The drawing under review shows one solid part. Ordinate dimensions are in mm from its lowest x, y, z. A direction names the side the tool comes from. Round coordinates to 2 decimals unless told otherwise and drop trailing zeros. Write each loop counter-clockwise with the first axis right and the second up, starting at its lowest first coordinate (ties: lowest second). Pieces come first, ordered by that corner, then holes. Notation, with made-up numbers: M 41,35.5 L 47,35.5 A6 ccw 47,45.5 Z; hole C 37.25,-29.75 d3. An arc over 180 degrees is marked long. One line per item, written item: value. Start each with the question number.
1) Take a section at C-C, the plane y = 3. Write out the cut boundary in (x, z).
2) Mouldability with a two-part tool opening along Y and no side actions: class the marked faces 4, 5 and 6 as +Y half, -Y half, draft (parallel to the pull), parting line (faces both ways), or undercut.
3) Tool access review of the marked faces 1, 2 and 3: name each direction out of +Z, -Z, +X, -X, +Y, -Y from which nothing blocks a thin tool from reaching the whole face with its end or side.
4) For P1, Ø6.5, axis at x = 7, z = 3.5, coming from the +Y side; P2, Ø3, axis at x = 11.5, y = 5, coming from the +Z side, all flat-tipped, find the tip position at first contact; note any pin that passes through.
5) Take a section at D-D, the plane x = 2. Write out the cut boundary in (y, z).
6) Take a section at B-B, the plane z = 3. Write out the cut boundary in (x, y), and give its area (3 significant figures).
7) Wall thickness on probe 1 along X at (y, z) = (0.35, 3); probe 2 along Z at (x, y) = (16, 1.05); probe 3 along X at (y, z) = (4.4, 12.25): over which ranges is each line inside the solid? List them lowest first.
8) Take a section at A-A, the plane x = 4. Write out the cut boundary in (y, z), and give its area (3 significant figures).
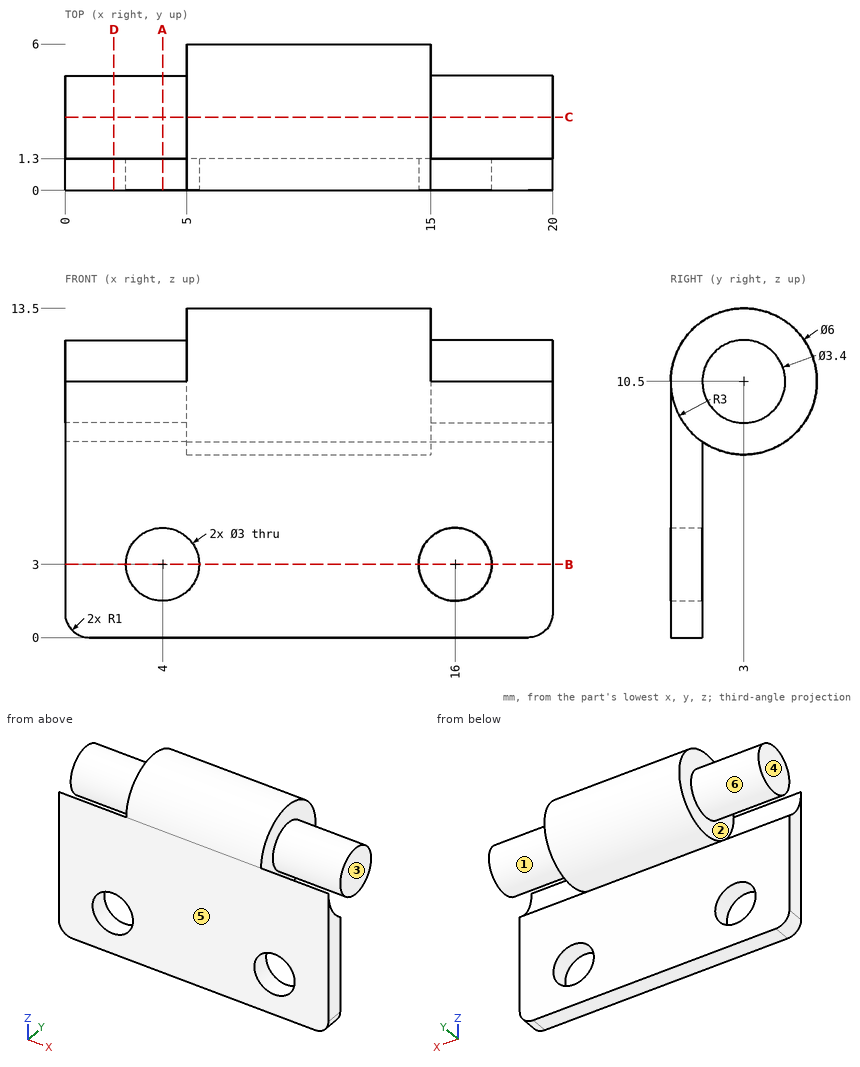
Checked values:
1. outline: M 0,8.8 L 5,8.8 L 5,7.5 L 15,7.5 L 15,8.8 L 20,8.8 L 20,12.2 L 15,12.2 L 15,13.5 L 5,13.5 L 5,12.2 L 0,12.2 Z
2. face 4: draft
2. face 5: -Y half
2. face 6: undercut
3. face 1: +X
3. face 2: -X
3. face 3: +Z, -Z, +X, +Y, -Y
4. P1: stops at y = 1.3
4. P2: stops at z = 13.46
5. outline: M 0,0 L 1.3,0 L 1.3,8.03 A3 cw 0,10.5 Z; C 3,10.5 d3.4
6. outline: M 0,0 L 2.5,0 L 2.5,1.3 L 0,1.3 Z; M 5.5,0 L 14.5,0 L 14.5,1.3 L 5.5,1.3 Z; M 17.5,0 L 20,0 L 20,1.3 L 17.5,1.3 Z
6. area: 18.2 mm2
7. probe 1: x = 0 to 2.5, 5.5 to 14.5, 17.5 to 20
7. probe 2: z = 0 to 1.5, 4.5 to 8.22
7. probe 3: x = 5 to 15
8. outline: M 0,0 L 1.3,0 L 1.3,1.5 L 0,1.5 Z; M 0,4.5 L 1.3,4.5 L 1.3,8.03 A3 cw 0,10.5 Z; C 3,10.5 d3.4
8. area: 16.6 mm2
